Answer from the drawing. Dimensions are ordinates in mm from the lowest x, y and z of the part. Round coordinates to 2 decimals unless told otherwise and drop trailing zeros. Order: outer loops, then holes, each group sorted by start corner. A loop starts at its lowest first (then second) coordinate and runs counter-clockwise, first axis right, second up. Notation, with made-up numbers: (-34, 19.25) - (5, 19.25) arc R28 ccw to (5, 58.25) - close; hole circle Ø10 at (26.5, -24). An arc over 180 degrees is marked (long way). One line per question, with ' | ' between items. Start each with the question number.
1) Flat-ended cylindrical pins translate along their axes: pin 1 (11 mm diameter, centred on x = 204, z = 3.5, fed in from -Y); pin 2 (12.5 mm diameter, centred on y = 35, z = 13.5, fed in from -X); pin 3 (12.5 mm diameter, centred on y = 39, z = 88, fed in from +X). Find the tip coordinate at first contact, or state that the pin passes through.
2) The mould has two halves that part along Z. Classify the marked faces 1 and 2: pulls with the +Z half, pulls with the -Z half, needs draft (parallel to the pull), parting line crosses it, or undercut.
3) The part is cut by section C-C, the plane y = 45. Give the vertices of the cut face in (x, z), plus the area to 3 significant figures.
4) The part is cut by section A-A, the plane y = 5.5. Give the vertices of the cut face in (x, z), plus the area to 3 significant figures.
5) The part is cut by section B-B, the plane x = 167.5. Give the vertices of the cut face in (y, z).
6) Straight lines are drawn through the part: line 1 (Y direction, x = 242, z = 21.5); line 2 (Y direction, x = 130, z = 38); line 3 (Z direction, x = 35, y = 45.5). For each, find the intervals that lie inside material, in ascending order. Write a range as from..to.
7) The part is cut by section D-D, the plane z = 22. Give the vertices of the cut face in (x, y).
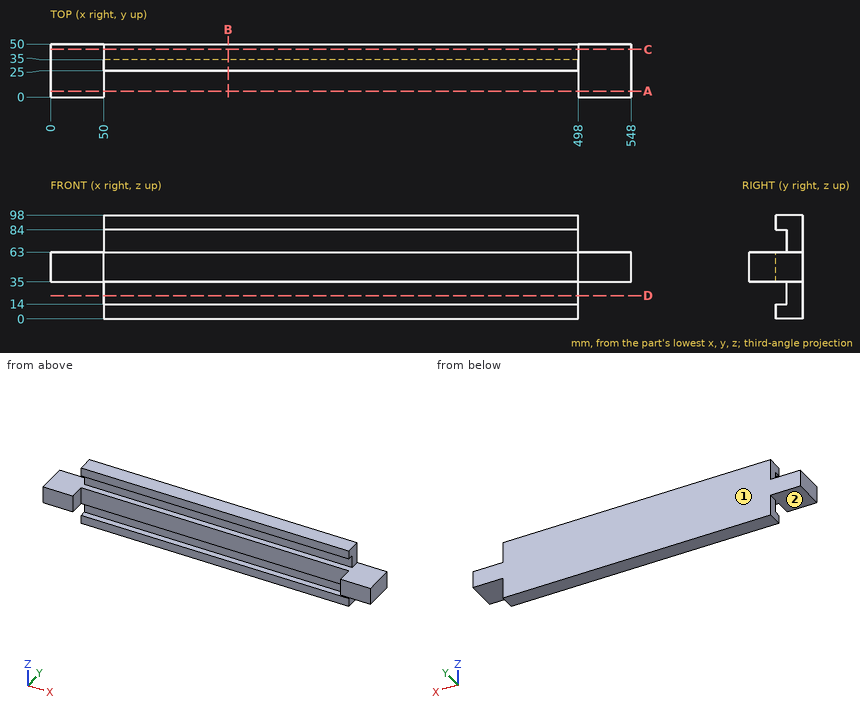
Values:
1) pin 1: stops at y = 25 | pin 2: stops at x = 50 | pin 3: stops at x = 498
2) face 1: needs draft | face 2: undercut
3) outline: (0, 35) - (50, 35) - (50, 0) - (498, 0) - (498, 35) - (548, 35) - (548, 63) - (498, 63) - (498, 98) - (50, 98) - (50, 63) - (0, 63) - close | area: 46,700 mm^2
4) outline: (0, 35) - (50, 35) - (50, 63) - (0, 63) - close; (498, 35) - (548, 35) - (548, 63) - (498, 63) - close | area: 2,800 mm^2
5) outline: (25, 0) - (50, 0) - (50, 98) - (25, 98) - (25, 84) - (35, 84) - (35, 63) - (25, 63) - (25, 35) - (35, 35) - (35, 14) - (25, 14) - close
6) line 1: y = 35..50 | line 2: y = 25..50 | line 3: z = 35..63
7) outline: (50, 35) - (498, 35) - (498, 50) - (50, 50) - close
